Print and shaded views of the part. All mm, measured from the part's lowest x, y and z. A direction names the side the tool comes from. Round coordinates to 2 decimals unless told otherwise and drop trailing zeros. Write each loop counter-clockwise with the first axis right and the second up, starting at its lowest first coordinate (ties: lowest second). Pieces come first, ordered by that corner, then holes.
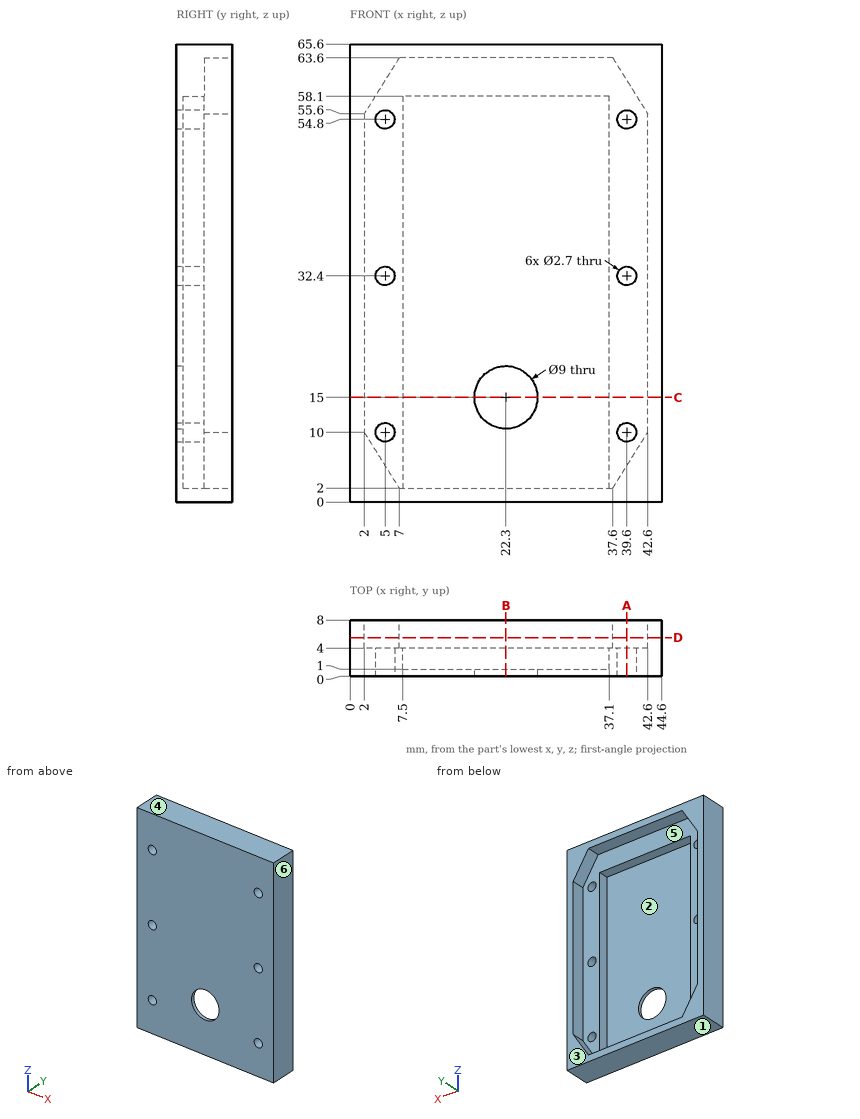
1) Mould opens along Z. For the marked faces 1, 2, 3 and 4 say: released by +Z, released by -Z, zero draft, split by the parting line, or undercut.
Results:
face 1: released by -Z
face 2: undercut
face 3: zero draft
face 4: released by +Z
2) Slice it at C-C (z = 15). Write the cut outline in (x, y).
Results:
outline: (0, 0) - (17.8, 0) - (17.8, 1) - (7.5, 1) - (7.5, 4) - (2, 4) - (2, 8) - (0, 8) - close; (26.8, 0) - (44.6, 0) - (44.6, 8) - (42.6, 8) - (42.6, 4) - (37.1, 4) - (37.1, 1) - (26.8, 1) - close
3) Slice it at A-A (x = 39.6). Write the cut outline in (y, z).
Results:
outline: (0, 0) - (8, 0) - (8, 5.2) - (4, 5.2) - (4, 8.65) - (0, 8.65) - close; (0, 11.35) - (4, 11.35) - (4, 31.05) - (0, 31.05) - close; (0, 33.75) - (4, 33.75) - (4, 53.45) - (0, 53.45) - close; (0, 56.15) - (4, 56.15) - (4, 60.4) - (8, 60.4) - (8, 65.6) - (0, 65.6) - close
4) Slice it at D-D (y = 5.5). Write the cut outline in (x, z).
Results:
outline: (0, 0) - (44.6, 0) - (44.6, 65.6) - (0, 65.6) - close; hole (2, 10) - (7, 2) - (37.6, 2) - (42.6, 10) - (42.6, 55.6) - (37.6, 63.6) - (7, 63.6) - (2, 55.6) - close
5) Pin check, flat tips, straight feed: pin 1 Ø1 at (x, z) = (26, 32) entering from +Y; pin 2 Ø1 at (x, z) = (38, 26.5) entering from +Y. Stop position of each tip, or through.
Results:
pin 1: stops at y = 1
pin 2: stops at y = 4
6) Which spindle directions (+Z, -Z, +X, -X, +Y, -Y) get a long thin tool onto all of the face, cutting with end or side? Do the marked faces 5 and 6. Say none if no direction does.
Results:
face 5: +Y
face 6: +Z, -Z, +X, +Y, -Y
7) Slice it at B-B (x = 22.3). Write the cut outline in (y, z), plus the area to 3 significant figures.
Results:
outline: (0, 0) - (8, 0) - (8, 2) - (1, 2) - (1, 10.5) - (0, 10.5) - close; (0, 19.5) - (1, 19.5) - (1, 58.1) - (4, 58.1) - (4, 63.6) - (8, 63.6) - (8, 65.6) - (0, 65.6) - close
area: 101 mm2
8) Wall check: L1, parallel to Z at x = 39.6, y = 2.15; L2, parallel to X at y = 2.45, z = 54.8; L3, parallel to Z at x = 13.5, y = 6.5. Give the ranges that are in metal, low to high.
Results:
L1: z = 0 to 8.65, 11.35 to 31.05, 33.75 to 53.45, 56.15 to 65.6
L2: x = 0 to 3.65, 6.35 to 7.5, 37.1 to 38.25, 40.95 to 44.6
L3: z = 0 to 2, 63.6 to 65.6
